The listing builds one solid part. Answer for the finished solid, in the listing's coordinates (mm). Face numbers are marked on the shaded views. A direction names the side the tool comes from. Give positions to 0.01 mm unless a question says otherwise; leave off trailing zeros. Loops run counter-clockwise (first coordinate to the right, second up) from the corner with the lowest first, then second, coordinate; pieces in that order, holes last. Notation, with made-up numbers: (47.25, 5) - (73.25, 5) arc R11 cw to (73.25, 15) - close; hole circle Ø6 at (26.5, 50). An arc over 180 degrees is marked (long way). Write item = value, one per line. Start each with the question number.
1) The part is cut by section D-D on y = 47. Write down the section's boundary in (x, z), plus the area to 3 significant figures.
2) Which of the six approach directions +Z, -Z, +X, -X, +Y, -Y give full straight-line access (tool end or side, diameter ignored) to the marked faces 4 and 5?
3) The mould has two halves that part along Z. Classify the marked faces 1, 2 and 3: +Z half, -Z half, draft (parallel to the pull), parting line (faces both ways), or undercut.
4) Flat-ended cylindrical pins translate along their axes: P1, Ø6, axis at y = -37.5, z = -31, coming from the +X side; P2, Ø3, axis at y = 49, z = -21.5, coming from the +X side; P3, Ø12, axis at x = 52, y = -43.5, coming from the +Z side; P4, Ø8, axis at x = -5, z = -38, coming from the -Y side. Find the tip coordinate at first contact, or state that the pin passes through.
5) The part is cut by section B-B on y = 27. Write down the section's boundary in (x, z).
6) The part is cut by section C-C on z = 0. Write down the section's boundary in (x, y) (3 decimals), plus the area to 3 significant figures.
7) Consider probe 1 along X at (y, z) = (-2.5, 13.5); probe 2 along Y at (x, z) = (57, -13.5); probe 3 along X at (y, z) = (-20, -7.5). Determine where each line is inside the solid, lowest interval first.
8) The part is cut by section A-A on x = 0. Write down the section's boundary in (y, z).
from build123d import *

# Parameters (mm, degrees)
SKETCH1_R                = 50
BOSS_EXTRUDE1_DEPTH      = 50
BOSS_EXTRUDE2_REACH      = 202.534
BOSS_EXTRUDE2_END_RADIUS = 65
SKETCH2_R                = 38.535
SKETCH2_R_2              = 38.035
BOSS_EXTRUDE3_START      = 3
SKETCH4_R                = 38.035
BOSS_EXTRUDE3_DEPTH      = 3


with BuildPart() as part:
    # Sketch1 → Boss-Extrude1 (new, symmetric)
    with BuildSketch(Plane.XY):
        with BuildLine():
            Line((-80, 40), (-80, -40))
            Line((-80, -40), (-22.281665693, -61.061668614))
            ThreePointArc((-22.281665693, -61.061668614), (65, 0), (-22.281665693, 61.061668614))
            Line((-22.281665693, 61.061668614), (-80, 40))
        make_face()
        Circle(SKETCH1_R, mode=Mode.SUBTRACT)
    extrude(amount=BOSS_EXTRUDE1_DEPTH, both=True)

    # Boss-Extrude2: up to this cylinder (the profile starts outside it)
    boss_extrude2_end = Plane(origin=(0, 0, 38.426007), z_dir=(0, 0, -1)) * Cylinder(BOSS_EXTRUDE2_END_RADIUS, 536.068, mode=Mode.PRIVATE)
    # Sketch2 → Boss-Extrude2 (add, up to the surface)
    with BuildSketch(Plane(origin=(103, 0, 0), x_dir=(0, 0, -1), z_dir=(1, 0, 0)), mode=Mode.PRIVATE) as boss_extrude2_sk1:
        Circle(SKETCH2_R)
        Circle(SKETCH2_R_2, mode=Mode.SUBTRACT)
    boss_extrude2_tool1 = extrude(boss_extrude2_sk1.sketch, amount=-BOSS_EXTRUDE2_REACH, mode=Mode.PRIVATE) - boss_extrude2_end
    add(boss_extrude2_tool1.solids().sort_by_distance((103, 0, 38.426007))[0])

    # Sketch4 → Boss-Extrude3 (add)
    with BuildSketch(Plane(origin=(68, 0, 0), x_dir=(0, 0, -1), z_dir=(1, 0, 0)).offset(BOSS_EXTRUDE3_START)):
        Circle(SKETCH4_R)
    extrude(amount=-BOSS_EXTRUDE3_DEPTH)


solid = part.part
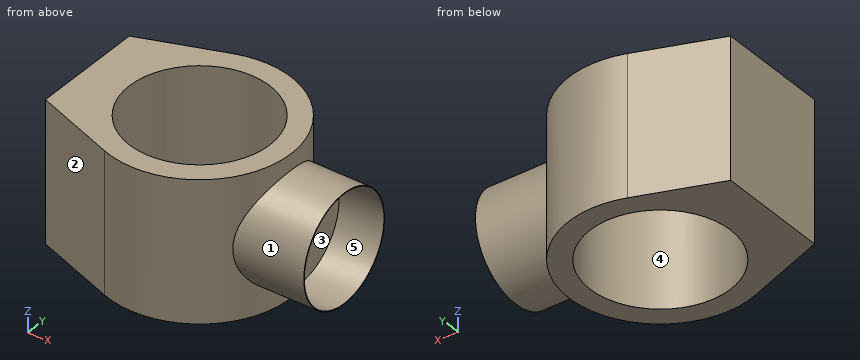
Answer below:
q1.outline = (-60.82, -50) - (-17.06, -50) - (-17.06, 50) - (-60.82, 50) - close; (17.06, -50) - (44.9, -50) - (44.9, 50) - (17.06, 50) - close
q1.area = 7,160 mm2
q2.face_4 = +Z, -Z
q2.face_5 = +X
q3.face_1 = parting line
q3.face_2 = draft
q3.face_3 = undercut
q4.P1 = 55.09
q4.P2 = 44.37
q4.P3 = 50
q4.P4 = -64.99
q5.outline = (-80, -50) - (-42.08, -50) - (-42.08, 50) - (-80, 50) - close; (42.08, -50) - (59.13, -50) - (59.13, -27.49) - (103, -27.49) - (103, -26.79) - (71, -26.79) - (71, 26.79) - (103, 26.79) - (103, 27.49) - (59.13, 27.49) - (59.13, 50) - (42.08, 50) - close; hole (59.13, -26.79) - (68, -26.79) - (68, 26.79) - (59.13, 26.79) - close
q6.outline = (-80, -40) - (-22.282, -61.062) arc R65 ccw to (52.346, -38.535) - (103, -38.535) - (103, -38.035) - (71, -38.035) - (71, 38.035) - (103, 38.035) - (103, 38.535) - (52.346, 38.535) arc R65 ccw to (-22.282, 61.062) - (-80, 40) - close; hole circle Ø100 at (0, 0); hole (52.71, -38.035) - (68, -38.035) - (68, 38.035) - (52.71, 38.035) arc R65 cw to start
q6.area = 7,730 mm2
q7.probe_1 = -80 to -49.94, 49.94 to 64.95, 68 to 71
q7.probe_2 = -36.09 to -35.56, -31.24 to 31.24, 35.56 to 36.09
q7.probe_3 = -80 to -45.83, 45.83 to 61.85, 68 to 71
q8.outline = (-65, -50) - (-50, -50) - (-50, 50) - (-65, 50) - close; (50, -50) - (65, -50) - (65, 50) - (50, 50) - close
